For this review, take the finished solid that the model builds, in its own axes (mm). A direction names the side the tool comes from. Give positions to 0.01 mm unless a question says otherwise; leave off trailing zeros. Write each loop counter-clockwise with the first axis right and the second up, starting at its lowest first coordinate (ties: lowest second). Pieces come first, ordered by that corner, then holes. Notation, with made-up numbers: M 45.5,42 L 66.5,42 A24 ccw 66.5,78 Z; hole C -14.75,73 d4. An arc over 180 degrees is marked long. Write item = value, one per line.
```python
from build123d import *

# Parameters (mm, degrees)
F1_DEPTH = 600


with BuildPart() as f1:
    # F0 (on Front) → F1 (new body)
    with BuildSketch(Plane.XZ):
        with BuildLine():
            Line((0, 75), (0, 0))
            Line((0, 0), (37.5, 0))
            ThreePointArc((37.5, 0), (39.267767, 0.732233), (40, 2.5))
            ThreePointArc((40, 2.5), (39.267767, 4.267767), (37.5, 5))
            Line((37.5, 5), (5, 5))
            Line((5, 5), (5, 70))
            Line((5, 70), (37.5, 70))
            ThreePointArc((37.5, 70), (39.267767, 70.732233), (40, 72.5))
            ThreePointArc((40, 72.5), (39.267767, 74.267767), (37.5, 75))
            Line((37.5, 75), (0, 75))
        make_face()
    extrude(amount=F1_DEPTH)


solid = f1.part
```
1. The part is to be moulded in two halves that separate along Z. For faces 1 (the face through (18, -296, 0)), 2 (the face through (4, 0, 38)), 3 (the face through (5, -296, 37)), say which applies: +Z half, -Z half, draft (parallel to the pull), parting line (faces both ways), or undercut.
Responses:
face_1 = -Z half
face_2 = draft
face_3 = undercut
2. We need section C-C, the plane z = 58. Write out the cut boundary in (x, y), then the cut area to 3 significant figures.
Responses:
outline = M 0,-600 L 5,-600 L 5,0 L 0,0 Z
area = 3,000 mm2
3. We need section B-B, the plane y = -110. Write out the cut boundary in (x, z), then the cut area to 3 significant figures.
Responses:
outline = M 0,0 L 37.5,0 A2.5 ccw 37.5,5 L 5,5 L 5,70 L 37.5,70 A2.5 ccw 37.5,75 L 0,75 Z
area = 720 mm2
4. Machinability: for faces 4 (the face through (21, -296, 5)), 5 (the face through (0, -296, 38)), which of the approach directions +Z, -Z, +X, -X, +Y, -Y give a long, thin tool a straight path to every point of the face, cutting with its end or side? Answer none if there is none.
Responses:
face_4 = +X, +Y, -Y
face_5 = +Z, -Z, -X, +Y, -Y
5. We need section A-A, the plane x = 31. Write out the cut boundary in (y, z), then the cut area to 3 significant figures.
Responses:
outline = M -600,0 L 0,0 L 0,5 L -600,5 Z; M -600,70 L 0,70 L 0,75 L -600,75 Z
area = 6,000 mm2
6. Insertion check: P1, Ø4, axis at y = -450.5, z = 63, coming from the +X side. The pin has a flat end and moves straight along its axis. Give the tip position at first contact, or say it passes through.
Responses:
P1 = 5
7. For line 1 along Z through (x, y) = (10.5, -399); line 2 along X through (y, z) = (-262, 47), list the stretches that pass through material, from the lowest coordinate up. Write a range as from..to.
Responses:
line_1 = 0..5, 70..75
line_2 = 0..5
